```python
from build123d import *

# Parameters (mm, degrees)
SKETCH1_R           = 4.8895
BOSS_EXTRUDE1_DEPTH = 3.937
BOSS_EXTRUDE2_DEPTH = 7.874
SKETCH3_R           = 5.08
BOSS_EXTRUDE3_DEPTH = 4.572
SKETCH4_R           = 6.223
BOSS_EXTRUDE4_DEPTH = 6.223
BOSS_EXTRUDE5_DEPTH = 5.969
SKETCH6_R           = 6.2865
BOSS_EXTRUDE6_DEPTH = 6.731
SKETCH7_R           = 5.2705
BOSS_EXTRUDE7_DEPTH = 4.318
SKETCH9_W           = 10.922
SKETCH9_H           = 10.922
BOSS_EXTRUDE8_DEPTH = 6.477
SKETCH10_R          = 20.955
BOSS_EXTRUDE9_DEPTH = 11.938
SKETCH11_R          = 3.18135
CUT_EXTRUDE1_DEPTH  = 11.938


with BuildPart() as part:
    # Sketch1 → Boss-Extrude1 (new body)
    with BuildSketch(Plane(origin=(0, 0, 0), x_dir=(1, 0, 0), z_dir=(0, 1, 0))):
        with Locations(Location((0, 0, 0), (0, 0, 270))):
            Circle(SKETCH1_R)
    extrude(amount=BOSS_EXTRUDE1_DEPTH)

    # Sketch2 → Boss-Extrude2 (add)
    with BuildSketch(Plane(origin=(0, 3.937, 0), x_dir=(1, 0, 0), z_dir=(0, 1, 0))):
        Polygon((7.772289324, 0), (3.886144662, 6.731), (-3.886144662, 6.731), (-7.772289324, 0), (-3.886144662, -6.731), (3.886144662, -6.731), align=None)
    extrude(amount=BOSS_EXTRUDE2_DEPTH)

    # Sketch3 → Boss-Extrude3 (add)
    with BuildSketch(Plane(origin=(0, 11.811, 0), x_dir=(1, 0, 0), z_dir=(0, 1, 0))):
        with Locations(Location((0, 0, 0), (0, 0, 270))):
            Circle(SKETCH3_R)
    extrude(amount=BOSS_EXTRUDE3_DEPTH)

    # Sketch4 → Boss-Extrude4 (add)
    with BuildSketch(Plane(origin=(0, 16.383, 0), x_dir=(1, 0, 0), z_dir=(0, 1, 0))):
        with Locations(Location((0, 0, 0), (0, 0, 270))):
            Circle(SKETCH4_R)
    extrude(amount=BOSS_EXTRUDE4_DEPTH)

    # Sketch5 → Boss-Extrude5 (add)
    with BuildSketch(Plane(origin=(0, 22.606, 0), x_dir=(1, 0, 0), z_dir=(0, 1, 0))):
        Polygon((7.332348419, 0), (3.666174209, 6.35), (-3.666174209, 6.35), (-7.332348419, 0), (-3.666174209, -6.35), (3.666174209, -6.35), align=None)
    extrude(amount=BOSS_EXTRUDE5_DEPTH)

    # Sketch6 → Boss-Extrude6 (add)
    with BuildSketch(Plane(origin=(0, 28.575, 0), x_dir=(1, 0, 0), z_dir=(0, 1, 0))):
        with Locations(Location((0, 0, 0), (0, 0, 270))):
            Circle(SKETCH6_R)
    extrude(amount=BOSS_EXTRUDE6_DEPTH)

    # Sketch7 → Boss-Extrude7 (add)
    with BuildSketch(Plane(origin=(0, 35.306, 0), x_dir=(1, 0, 0), z_dir=(0, 1, 0))):
        with Locations(Location((0, 0, 0), (0, 0, 270))):
            Circle(SKETCH7_R)
    extrude(amount=BOSS_EXTRUDE7_DEPTH)

    # Sketch9 → Boss-Extrude8 (add)
    with BuildSketch(Plane(origin=(0, 39.624, 0), x_dir=(1, 0, 0), z_dir=(0, 1, 0))):
        Rectangle(SKETCH9_W, SKETCH9_H)
    extrude(amount=BOSS_EXTRUDE8_DEPTH)

    # Sketch10 → Boss-Extrude9 (add)
    with BuildSketch(Plane(origin=(0, 46.101, 0), x_dir=(1, 0, 0), z_dir=(0, 1, 0))):
        with Locations(Location((0, 0, 0), (0, 0, 270))):
            Circle(SKETCH10_R)
    extrude(amount=BOSS_EXTRUDE9_DEPTH)

    # Sketch11 → Cut-Extrude1 (cut)
    with BuildSketch(Plane.XZ):
        with Locations(Location((0, 0, 0), (0, 0, 270))):
            Circle(SKETCH11_R)
    extrude(amount=-CUT_EXTRUDE1_DEPTH, mode=Mode.SUBTRACT)


solid = part.part
```
The model under review builds one solid part; all positions refer to its coordinate system, in mm. A direction names the side the tool comes from. Give positions to 0.01 mm unless a question says otherwise; leave off trailing zeros. Write each loop counter-clockwise with the first axis right and the second up, starting at its lowest first coordinate (ties: lowest second). Pieces come first, ordered by that corner, then holes. Notation, with made-up numbers: (25, 61) - (48, 61) arc R22 cw to (48, 92) - close; hole circle Ø7 at (70.25, 68.5). An arc over 180 degrees is marked (long way). Answer in a Markdown table with one row per item. Add a question column.
1. We need section C-C on y = 52. Write out the cut boundary in (x, z) (3 decimals), then the cut area to 3 significant figures.
2. We need section B-B on z = 12.5. Write out the cut boundary in (x, y).
3. We need section D-D on z = -7.5. Write out the cut boundary in (x, y), then the cut area to 3 significant figures.
4. Draft analysis for pull direction Y (two halves, no side actions). For faces 6 (the flat face through (-1, 0, 3.2)), 7 (the flat face through (-5.474, 25.549, -3.219)), 8 (the cylindrical face through (17.669, 51.986, 11.265)), state which applies: +Y half, -Y half, draft (parallel to the pull), parting line (faces both ways), or undercut.
5. We need section A-A on y = 31. Write out the cut boundary in (x, z), then the cut area to 3 significant figures.
6. Wall thickness on line 1 along X through (y, z) = (7.25, 0); line 2 along Y through (x, z) = (9, 12); line 3 along X through (y, z) = (3.5, 0): over which ranges is each line inside the solid? List them lowest first. Write a range as [from, to].
7. Insertion check: P1, Ø5, axis at y = 41.5, z = 0, coming from the -X side; P2, Ø12, axis at x = 14.5, y = 47, coming from the +Z side; P3, Ø1, axis at y = 51.5, z = 14.5, coming from the -X side. Each pin has a flat end and moves straight along its axis. Give the tip position at first contact, or say it passes through.
8. Tool access review of faces 1 (the flat face through (0, 43, 5.461)), 2 (the flat face through (0, 8, -6.731)), 3 (the flat face through (5.525, 25.549, -3.131)), 4 (the flat face through (0, 26, -6.35)), 5 (the flat face through (-5.802, 7.819, -3.413)): name each direction out of +Z, -Z, +X, -X, +Y, -Y from which nothing blocks a thin tool from reaching the whole face with its end or side.
Ans:
| question | item | result |
|---|---|---|
| 1 | outline | circle Ø41.91 at (0, 0) |
| 1 | area | 1,380 mm^2 |
| 2 | outline | (-16.82, 46.1) - (16.82, 46.1) - (16.82, 58.04) - (-16.82, 58.04) - close |
| 3 | outline | (-19.57, 46.1) - (19.57, 46.1) - (19.57, 58.04) - (-19.57, 58.04) - close |
| 3 | area | 467 mm^2 |
| 4 | face 6 | -Y half |
| 4 | face 7 | undercut |
| 4 | face 8 | draft |
| 5 | outline | circle Ø12.57 at (0, 0) |
| 5 | area | 124 mm^2 |
| 6 | line 1 | x = [-7.77, -3.18], [3.18, 7.77] |
| 6 | line 2 | y = [46.1, 58.04] |
| 6 | line 3 | x = [-4.89, -3.18], [3.18, 4.89] |
| 7 | P1 | stops at x = -5.46 |
| 7 | P2 | stops at z = 19.15 |
| 7 | P3 | stops at x = -15.59 |
| 8 | face 1 | +Z, +X, -X |
| 8 | face 2 | -Z, +X, -X, -Y |
| 8 | face 3 | -Z, +X |
| 8 | face 4 | -Z, +X, -X |
| 8 | face 5 | -Z, -X, -Y |
